Geometry check sheet. Reference: the model listing, model coordinates, mm. A direction names the side the tool comes from. Round coordinates to 2 decimals unless told otherwise and drop trailing zeros. Order: outer loops, then holes, each group sorted by start corner. A loop starts at its lowest first (then second) coordinate and runs counter-clockwise, first axis right, second up. Notation, with made-up numbers: (38, -28.75) -> (65, -28.75) arc R15 ccw to (65, -17.75) -> close; hole circle Ø2 at (-27.5, 57.5). An arc over 180 degrees is marked (long way). Use a Markdown table: item, result. Add a question column.
Item 1: Mould release check, pull along X, two halves, no side actions. Record for faces 1 (the flat face through (16, 2, 4)), 2 (the flat face through (-14.48, -3.47, 4.44)), 3 (the cylindrical face through (-12.873, 2.12, 3.204)): pulls with the +X half, pulls with the -X half, needs draft (parallel to the pull), parting line crosses it, or undercut.
Item 2: Sectioned sample at D-D, the plane z = 1.5. Record the cut outline in (x, y).
Item 3: Set-up check for faces 4 (the flat face through (13.974, 2, 8)), 5 (the flat face through (-16, 2, 4)), 6 (the flat face through (0, 0.3, 4)): record each of +Z, -Z, +X, -X, +Y, -Y from which the full face is reachable in a straight line by a thin tool's end or side.
Item 4: Sectioned sample at B-B, the plane z = 7.5. Record the cut outline in (x, y).
Item 5: Gauge pin test, flat ends, axial feed: pin 1 Ø8 at (x, y) = (12.5, 1.5) entering from -Z; pin 2 Ø3 at (x, y) = (11.27, 2.05) entering from -Z; pin 3 Ø1.6 at (x, y) = (-11, 3.5) entering from +Z. Record the tip position at first contact, or that the pin passes through.
Item 6: Material ranges on probe 1 along X at (y, z) = (2.05, 4.75); probe 2 along Y at (x, z) = (2, 6.25); probe 3 along Y at (x, z) = (-12, 7.5), recorded low to high. Write a range as [from, to].
Item 7: Sectioned sample at C-C, the plane x = -4. Record the cut outline in (y, z).
Item 8: Sectioned sample at A-A, the plane y = 2.05. Record the cut outline in (x, z), and give its area (3 significant figures).
from build123d import *

# Parameters (mm, degrees)
F0_W     = 32
F0_H     = 14
F0_R     = 1.6
F0_W_2   = 9.6
F0_H_2   = 3.5
F1_DEPTH = 9
F2_SIZE  = 3
F4_DEPTH = 2.5


with BuildPart() as f1:
    # F0 (on Top) → F1 (new body)
    with BuildSketch(Plane.XY):
        with Locations((0, 2.05)):
            Rectangle(F0_W, F0_H)
        with Locations((-11.274233, 2.05)):
            Circle(F0_R, mode=Mode.SUBTRACT)
        with Locations((0, 2.05)):
            Rectangle(F0_W_2, F0_H_2, mode=Mode.SUBTRACT)
        with Locations((11.274233, 2.05)):
            Circle(F0_R, mode=Mode.SUBTRACT)
    extrude(amount=F1_DEPTH)

    # F2
    f2_edges = [f1.edges().sort_by_distance(p)[0] for p in [
        (-16, -4.95, 4.5),
        (16, -4.95, 4.5),
        (16, 9.05, 4.5),
        (-16, 9.05, 4.5),
    ]]
    chamfer(f2_edges, length=F2_SIZE)

    # F3 (on face) → F4 (cut)
    with BuildSketch(Plane.XY.offset(9)):
        Polygon((-8.574233, 0.491154), (-8.574233, 3.608846), (-11.274233, 5.167691), (-13.974233, 3.608846), (-13.974233, 0.491154), (-11.274233, -1.067691), align=None)
        Polygon((13.974233, 0.491154), (13.974233, 3.608846), (11.274233, 5.167691), (8.574233, 3.608846), (8.574233, 0.491154), (11.274233, -1.067691), align=None)
    extrude(amount=-F4_DEPTH, mode=Mode.SUBTRACT)


solid = f1.part
Found:
| question | item | result |
|---|---|---|
| 1 | face 1 | pulls with the +X half |
| 1 | face 2 | pulls with the -X half |
| 1 | face 3 | undercut |
| 2 | outline | (-16, -1.95) -> (-13, -4.95) -> (13, -4.95) -> (16, -1.95) -> (16, 6.05) -> (13, 9.05) -> (-13, 9.05) -> (-16, 6.05) -> close; hole circle Ø3.2 at (-11.27, 2.05); hole (-4.8, 0.3) -> (4.8, 0.3) -> (4.8, 3.8) -> (-4.8, 3.8) -> close; hole circle Ø3.2 at (11.27, 2.05) |
| 3 | face 4 | +Z |
| 3 | face 5 | +Z, -Z, -X, +Y, -Y |
| 3 | face 6 | +Z, -Z |
| 4 | outline | (-16, -1.95) -> (-13, -4.95) -> (13, -4.95) -> (16, -1.95) -> (16, 6.05) -> (13, 9.05) -> (-13, 9.05) -> (-16, 6.05) -> close; hole (-13.97, 0.49) -> (-11.27, -1.07) -> (-8.57, 0.49) -> (-8.57, 3.61) -> (-11.27, 5.17) -> (-13.97, 3.61) -> close; hole (-4.8, 0.3) -> (4.8, 0.3) -> (4.8, 3.8) -> (-4.8, 3.8) -> close; hole (8.57, 0.49) -> (11.27, -1.07) -> (13.97, 0.49) -> (13.97, 3.61) -> (11.27, 5.17) -> (8.57, 3.61) -> close |
| 5 | pin 1 | stops at z = 0 |
| 5 | pin 2 | passes through |
| 5 | pin 3 | stops at z = 6.5 |
| 6 | probe 1 | x = [-16, -12.87], [-9.67, -4.8], [4.8, 9.67], [12.87, 16] |
| 6 | probe 2 | y = [-4.95, 0.3], [3.8, 9.05] |
| 6 | probe 3 | y = [-4.95, -0.65], [4.75, 9.05] |
| 7 | outline | (-4.95, 0) -> (0.3, 0) -> (0.3, 9) -> (-4.95, 9) -> close; (3.8, 0) -> (9.05, 0) -> (9.05, 9) -> (3.8, 9) -> close |
| 8 | outline | (-16, 0) -> (-12.87, 0) -> (-12.87, 6.5) -> (-13.97, 6.5) -> (-13.97, 9) -> (-16, 9) -> close; (-9.67, 0) -> (-4.8, 0) -> (-4.8, 9) -> (-8.57, 9) -> (-8.57, 6.5) -> (-9.67, 6.5) -> close; (4.8, 0) -> (9.67, 0) -> (9.67, 6.5) -> (8.57, 6.5) -> (8.57, 9) -> (4.8, 9) -> close; (12.87, 0) -> (16, 0) -> (16, 9) -> (13.97, 9) -> (13.97, 6.5) -> (12.87, 6.5) -> close |
| 8 | area | 133 mm2 |
